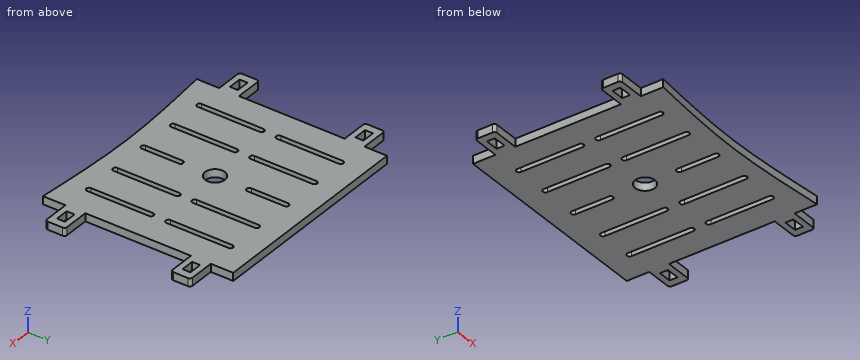
```python
from build123d import *

# Parameters (mm, degrees)
F1_W     = 21
F1_H     = 15
F2_DEPTH = 6
F0_R     = 7.5
F3_DEPTH = 25
F5_DEPTH = 25
F6_R     = 2
F7_W     = 10
F7_H     = 6
F8_DEPTH = 25


with BuildPart() as f2:
    # F1 (on Top) → F2 (new body)
    with BuildSketch(Plane.XY):
        Polygon((-80, -72), (80, -72), (80, -55), (80, -40), (80, 40), (80, 55), (80, 72), (-80, 72), (-80, 55), (-80, 40), (-80, -40), (-80, -55), align=None)
        with Locations((90.5, -47.5)):
            Rectangle(F1_W, F1_H)
        with Locations((-90.5, -47.5)):
            Rectangle(F1_W, F1_H)
        with Locations((90.5, 47.5)):
            Rectangle(F1_W, F1_H)
        with Locations((-90.5, 47.5)):
            Rectangle(F1_W, F1_H)
    extrude(amount=-F2_DEPTH)

    # F0 (on Top) → F3 (cut)
    with BuildSketch(Plane.XY):
        with BuildLine():
            ThreePointArc((-57.5, 55.5), (-58.9142135624, 54.9142135624), (-59.5, 53.5))
            Line((-59.5, 53.5), (-59.5, 6.5))
            ThreePointArc((-59.5, 6.5), (-58.9142135624, 5.0857864376), (-57.5, 4.5))
            ThreePointArc((-57.5, 4.5), (-56.0857864376, 5.0857864376), (-55.5, 6.5))
            Line((-55.5, 6.5), (-55.5, 53.5))
            ThreePointArc((-55.5, 53.5), (-56.0857864376, 54.9142135624), (-57.5, 55.5))
        make_face()
        with BuildLine():
            ThreePointArc((-59.5, -53.5), (-58.9142135624, -54.9142135624), (-57.5, -55.5))
            ThreePointArc((-57.5, -55.5), (-56.0857864376, -54.9142135624), (-55.5, -53.5))
            Line((-55.5, -53.5), (-55.5, -6.5))
            ThreePointArc((-55.5, -6.5), (-56.0857864376, -5.0857864376), (-57.5, -4.5))
            ThreePointArc((-57.5, -4.5), (-58.9142135624, -5.0857864376), (-59.5, -6.5))
            Line((-59.5, -6.5), (-59.5, -53.5))
        make_face()
        with BuildLine():
            ThreePointArc((-28, 53.5), (-28.5857864376, 54.9142135624), (-30, 55.5))
            ThreePointArc((-30, 55.5), (-31.4142135624, 54.9142135624), (-32, 53.5))
            Line((-32, 53.5), (-32, 6.5))
            ThreePointArc((-32, 6.5), (-31.4142135624, 5.0857864376), (-30, 4.5))
            ThreePointArc((-30, 4.5), (-28.5857864376, 5.0857864376), (-28, 6.5))
            Line((-28, 6.5), (-28, 53.5))
        make_face()
        with BuildLine():
            ThreePointArc((-28, -6.5), (-28.5857864376, -5.0857864376), (-30, -4.5))
            ThreePointArc((-30, -4.5), (-31.4142135624, -5.0857864376), (-32, -6.5))
            Line((-32, -6.5), (-32, -53.5))
            ThreePointArc((-32, -53.5), (-31.4142135624, -54.9142135624), (-30, -55.5))
            ThreePointArc((-30, -55.5), (-28.5857864376, -54.9142135624), (-28, -53.5))
            Line((-28, -53.5), (-28, -6.5))
        make_face()
        Circle(F0_R)
        with BuildLine():
            ThreePointArc((0, 24), (1.4142135624, 24.5857864376), (2, 26))
            Line((2, 26), (2, 54))
            ThreePointArc((2, 54), (1.4142135624, 55.4142135624), (0, 56))
            ThreePointArc((0, 56), (-1.4142135624, 55.4142135624), (-2, 54))
            Line((-2, 54), (-2, 26))
            ThreePointArc((-2, 26), (-1.4142135624, 24.5857864376), (0, 24))
        make_face()
        with BuildLine():
            Line((2, -54), (2, -26))
            ThreePointArc((2, -26), (1.4142135624, -24.5857864376), (0, -24))
            ThreePointArc((0, -24), (-1.4142135624, -24.5857864376), (-2, -26))
            Line((-2, -26), (-2, -54))
            ThreePointArc((-2, -54), (-1.4142135624, -55.4142135624), (0, -56))
            ThreePointArc((0, -56), (1.4142135624, -55.4142135624), (2, -54))
        make_face()
        with BuildLine():
            Line((28, -6.5), (28, -53.5))
            ThreePointArc((28, -53.5), (28.5857864376, -54.9142135624), (30, -55.5))
            ThreePointArc((30, -55.5), (31.4142135624, -54.9142135624), (32, -53.5))
            Line((32, -53.5), (32, -6.5))
            ThreePointArc((32, -6.5), (31.4142135624, -5.0857864376), (30, -4.5))
            ThreePointArc((30, -4.5), (28.5857864376, -5.0857864376), (28, -6.5))
        make_face()
        with BuildLine():
            ThreePointArc((30, 4.5), (31.4142135624, 5.0857864376), (32, 6.5))
            Line((32, 6.5), (32, 53.5))
            ThreePointArc((32, 53.5), (31.4142135624, 54.9142135624), (30, 55.5))
            ThreePointArc((30, 55.5), (28.5857864376, 54.9142135624), (28, 53.5))
            Line((28, 53.5), (28, 6.5))
            ThreePointArc((28, 6.5), (28.5857864376, 5.0857864376), (30, 4.5))
        make_face()
        with BuildLine():
            ThreePointArc((55.5, 6.5), (56.0857864376, 5.0857864376), (57.5, 4.5))
            ThreePointArc((57.5, 4.5), (58.9142135624, 5.0857864376), (59.5, 6.5))
            Line((59.5, 6.5), (59.5, 53.5))
            ThreePointArc((59.5, 53.5), (58.9142135624, 54.9142135624), (57.5, 55.5))
            ThreePointArc((57.5, 55.5), (56.0857864376, 54.9142135624), (55.5, 53.5))
            Line((55.5, 53.5), (55.5, 6.5))
        make_face()
        with BuildLine():
            ThreePointArc((55.5, -53.5), (56.0857864376, -54.9142135624), (57.5, -55.5))
            ThreePointArc((57.5, -55.5), (58.9142135624, -54.9142135624), (59.5, -53.5))
            Line((59.5, -53.5), (59.5, -6.5))
            ThreePointArc((59.5, -6.5), (58.9142135624, -5.0857864376), (57.5, -4.5))
            ThreePointArc((57.5, -4.5), (56.0857864376, -5.0857864376), (55.5, -6.5))
            Line((55.5, -6.5), (55.5, -53.5))
        make_face()
    extrude(amount=-F3_DEPTH, mode=Mode.SUBTRACT)

    # F4 (on face) → F5 (cut)
    with BuildSketch(Plane.XY):
        with BuildLine():
            add(Edge.make_bspline(
                [(-80, -72), (-53.3333333333, -69.4902703762), (0, -64.4708111286), (53.3333333333, -69.4902703762), (80, -72)],
                knots=[0, 0, 0, 0, 0.5, 1, 1, 1, 1], degree=3))
            Line((-80, -72), (-75.6795704365, -86.1006528139))
            Line((-75.6795704365, -86.1006528139), (77.3649588227, -86.1006528139))
            Line((77.3649588227, -86.1006528139), (80, -72))
        make_face()
    extrude(amount=-F5_DEPTH, mode=Mode.SUBTRACT)

    # F6
    f6_edges = [f2.edges().sort_by_distance(p)[0] for p in [
        (-101, 40, -3),
        (-101, 55, -3),
        (-101, -40, -3),
        (-101, -55, -3),
        (101, -55, -3),
        (101, -40, -3),
        (101, 40, -3),
        (101, 55, -3),
    ]]
    fillet(f6_edges, radius=F6_R)

    # F7 (on face) → F8 (cut)
    with BuildSketch(Plane.XY):
        with Locations((-90, 47.5)):
            Rectangle(F7_W, F7_H)
        with Locations((-90, -47.5)):
            Rectangle(F7_W, F7_H)
        with Locations((90, 47.5)):
            Rectangle(F7_W, F7_H)
        with Locations((90, -47.5)):
            Rectangle(F7_W, F7_H)
    extrude(amount=-F8_DEPTH, mode=Mode.SUBTRACT)


solid = f2.part
```
Can you work these out from the model? Positions are in its coordinate system, mm. Coordinates: 2 decimals unless noted, no trailing zeros. Loops run counter-clockwise (first coordinate to the right, second up) from the corner with the lowest first, then second, coordinate; pieces in that order, holes last. Notation, with made-up numbers: M -27.75,72.25 L 1.25,72.25 A6 ccw 1.25,77.25 Z; hole C 15.25,5 d8. An arc over 180 degrees is marked long. Put each result on its own line as item: value. Start each with the question number.
(1) Will these pins go through, and if not, where does the flat tip stop? pin 1 Ø3 at (y, z) = (-33, -2.5) entering from +X; pin 2 Ø3 at (x, z) = (-86.5, -2) entering from +Y; pin 3 Ø3 at (x, z) = (89.5, -2.5) entering from -Y; pin 4 Ø3 at (y, z) = (41.5, -2) entering from +X.
(2) Imagine slicing it at A-A on y = 0. List the corners of the cut face in (x, z) for me.
(3) I need wall thicknesses on probe 1 along X at (y, z) = (-52, -2); probe 2 along X at (y, z) = (39.5, -0.25); probe 3 along Y at (x, z) = (0.5, -2). Which ranges of each line are inside material? Lowest first, please.
(4) Imagine slicing it at B-B on y = 33. List the corners of the cut face in (x, z) for me, and give its area (3 significant figures).
(5) Imagine slicing it at C-C on z = -2.5. Give the number of separate pieces and of enclosed holes in the cut face, and give its area (3 significant figures).
Worked answers:
1. pin 1: stops at x = 80
1. pin 2: stops at y = 55
1. pin 3: stops at y = -55
1. pin 4: stops at x = 101
2. outline: M -80,-6 L -7.5,-6 L -7.5,0 L -80,0 Z; M 7.5,-6 L 80,-6 L 80,0 L 7.5,0 Z
3. probe 1: x = -101 to -59.5, -55.5 to -32, -28 to -2, 2 to 28, 32 to 55.5, 59.5 to 101
3. probe 2: x = -80 to -59.5, -55.5 to -32, -28 to -2, 2 to 28, 32 to 55.5, 59.5 to 80
3. probe 3: y = -66.98 to -55.94, -24.06 to -7.48, 7.48 to 24.06, 55.94 to 72
4. outline: M -80,-6 L -59.5,-6 L -59.5,0 L -80,0 Z; M -55.5,-6 L -32,-6 L -32,0 L -55.5,0 Z; M -28,-6 L -2,-6 L -2,0 L -28,0 Z; M 2,-6 L 28,-6 L 28,0 L 2,0 Z; M 32,-6 L 55.5,-6 L 55.5,0 L 32,0 Z; M 59.5,-6 L 80,-6 L 80,0 L 59.5,0 Z
4. area: 840 mm2
5. separate pieces: 1
5. enclosed holes: 15
5. area: 21,500 mm2
